For this review, take the finished solid that the model builds, in its own axes (mm). Face numbers are marked on the shaded views. A direction names the side the tool comes from. Round coordinates to 2 decimals unless told otherwise and drop trailing zeros. Order: outer loops, then holes, each group sorted by start corner. A loop starts at its lowest first (then second) coordinate and runs counter-clockwise, first axis right, second up. Notation, with made-up numbers: (-22.5, 55.5) - (13.5, 55.5) arc R34 ccw to (13.5, 85.5) - close; hole circle Ø10 at (33.5, 23.5). An arc over 180 degrees is marked (long way). One line per question, with ' | ' between items.
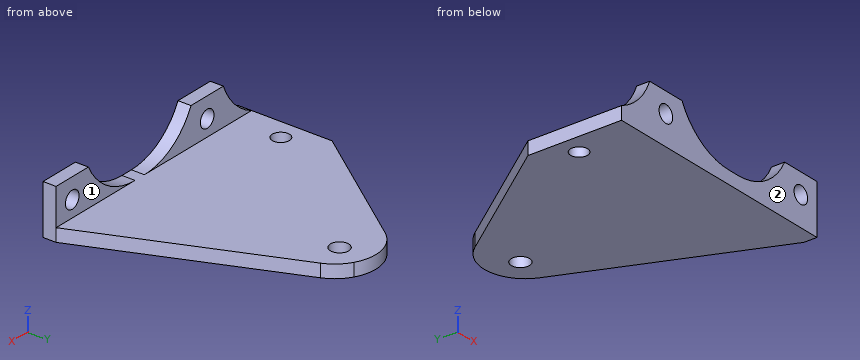
Autodesk Inventor part; units mm, degrees
ref_plane "YZ Plane" through (0, 0, 0) normal (1, 0, 0) x (0, 1, 0)
ref_plane "XZ Plane" through (0, 0, 0) normal (0, 1, 0) x (-1, 0, 0)
ref_plane "XY Plane" through (0, 0, 0) normal (0, 0, 1) x (1, 0, 0)
sketch "Эскиз1" plane through (0, 0, 0) normal (0, 0, 1) x (1, 0, 0)
  circle A0 centre (0, 0) radius 2.1
  line L0 (-5, 14.35) -> (5, 14.35)
  line L1 (5, 14.35) -> (5, -14.35)
  line L2 (5, -14.35) -> (-5, -14.35)
  line L3 (-5, -14.35) -> (-5, 14.35)
  line L4 (-5, 14.35) -> (5, -14.35) construction
  line L5 (5, 14.35) -> (-5, -14.35) construction
  line L6 (-5, 7) -> (5, 7)
  dimension "d0" = 4.2
  dimension "d2" = 10
  dimension "d3" = 28.7
  dimension "d4" = 7
extrude "Выдавливание1" add sketch "Эскиз1" along normal blind 3.2 contours L6 L1 L2 L3
sketch "Эскиз2" plane through (0, 0, 3.2) normal (0, 0, 1) x (1, 0, 0)
  line L0 (5, -14.35) -> (5, 7)
  line L1 (5, -14.35) -> (-5, -14.35)
  line L2 (-5, -14.35) -> (-5, -11.15)
  line L3 (-5, -11.15) -> (5, -11.15)
  line L4 (5, -11.15) -> (5, -14.35)
  point P0 (0, 0)
  point P1 (5, -11.15)
  dimension "d7" = 10
  dimension "d8" = 3.2
extrude "Выдавливание2" add sketch "Эскиз2" along normal blind 13
sketch "Эскиз3" plane through (-5, -11.15, 16.2) normal (0, 1, 0) x (1, 0, 0)
  line L0 (0, 10) -> (10, 10)
  line L1 (5, 10) -> (5, 0)
  line L2 (0, 0) -> (10, 0)
  circle A0 centre (5, 5) radius 2.1
  point P0 (5, 16.2)
  dimension "d12" = 4.2
extrude "Выдавливание3" cut sketch "Эскиз3" against normal blind 13
sketch "Эскиз4" plane through (0, 0, 3.2) normal (0, 0, 1) x (1, 0, 0)
  circle A0 centre (27.823512, 36.442015) radius 2.691667
  line L0 (25.598764, 34.926903) -> (0, 0)
  line L1 (17.757888, 39.624709) -> (-5, 8.573892)
  line L2 (-5, 7) -> (-5, -11.15)
  line L3 (-5, 7) -> (-5, 8.573892)
  line L4 (-5, -14.35) -> (5, -14.35)
  line L5 (5, -14.35) -> (5, -11.15)
  line L6 (5, -11.15) -> (-5, -11.15)
  line L7 (-5, -11.15) -> (-5, -14.35)
  line L8 (27.823512, 36.442015) -> (27.823512, -3.381482)
  line L9 (35.823512, 33.713219) -> (35.823512, -14.35)
  arc A1 (35.823512, 33.713219) -> (17.757888, 39.624709) centre (25.823512, 33.713219) ccw
  line L10 (-5, -14.35) -> (35.823512, -14.35)
  circle A2 centre (27.823512, 36.442015) radius 2.25
  line L11 (-5, 8.573892) -> (-5, -14.35)
  circle A3 centre (0, 0) radius 2.1
  point P0 (-5, -8.15)
  point P1 (-5, -11.15)
  dimension "d15" = 10
  dimension "d16" = 8
  dimension "d17" = 10
  dimension "d18" = 4.5
extrude "Выдавливание4" add sketch "Эскиз4" against normal up to surface (3.2 mm away) contours A0 | A1 L9 L10 L5 L6 L2 L3 L1
ref_plane "РабПлоскость1" through (20.202, -14.35, 16.2) normal (-1, 0, 0) x (0, 0, 1)
mirror "Зеркальное отражение1" about plane through (20.202, -14.35, 16.2) normal (-1, 0, 0) of "Выдавливание2", "Выдавливание3"
sketch "Эскиз6" plane through (0, 0, 0) normal (0, 0, -1) x (-1, 0, 0)
  circle A0 centre (-17.823512, 36.442015) radius 2.25
  circle A1 centre (10, 0) radius 2.1
  line L0 (5, -14.35) -> (-35.823512, -14.35)
  line L1 (5, -14.35) -> (5, 8.573892)
  line L2 (15, 8.573892) -> (-7.757888, 39.624709)
  arc A2 (-7.757888, 39.624709) -> (-25.823512, 33.713219) centre (-15.823512, 33.713219) ccw
  line L3 (-25.823512, 33.713219) -> (-25.823512, -14.35)
  circle A3 centre (-27.823512, 36.442015) radius 2.25
  circle A4 centre (0, 0) radius 2.1
  line L4 (5, -14.35) -> (-35.823512, -14.35)
  line L5 (5, -14.35) -> (5, 8.573892)
  line L6 (5, 8.573892) -> (-17.757888, 39.624709)
  arc A5 (-17.757888, 39.624709) -> (-35.823512, 33.713219) centre (-25.823512, 33.713219) ccw
  line L7 (-35.823512, 33.713219) -> (-35.823512, -14.35)
  line L8 (-35.823512, -14.35) -> (-35.823512, -11.15)
  line L9 (-35.823512, -11.15) -> (-45.404, -11.15)
  line L10 (-45.404, -11.15) -> (-45.404, -14.35)
  line L11 (-45.404, -14.35) -> (-35.823512, -14.35)
  line L12 (-25.823512, -14.35) -> (-45.404, -14.35)
  line L13 (0, 0) -> (10, 0)
  line L14 (15, 8.573892) -> (15, -18.0489)
  line L15 (-5, -14.35) -> (-35.404, -14.35)
  line L16 (-8, -14.35) -> (16.577235, -14.35)
  line L17 (-45.404, -11.15) -> (-35.708646, 35.224555)
  point P0 (-10, 0)
  point P1 (-20.823512, 42.373473)
  point P2 (15, -14.35)
  point P3 (-16.942673, 38.512431)
  point P4 (-15.583961, 36.658607)
  point P5 (5, 8.573892)
  dimension "d35" = 10
extrude "Выдавливание5" add sketch "Эскиз6" against normal up to surface (3.2 mm away) contours A0 L6 A5 A2 L2 L14 L16 L1 | A5 L7 L9 L17 | L9 L7 L11 L10
extrude "Выдавливание6" cut sketch "Эскиз6" against normal blind 10 contours A0 L6 | L6 A0 | A1
sketch "Эскиз7" plane through (0, 0, 3.2) normal (0, 0, 1) x (1, 0, 0)
  circle A0 centre (0, 0) radius 2.1
  line L0 (35.404, -14.35) -> (35.404, -11.15)
  line L1 (5, -14.35) -> (35.404, -14.35)
  arc A1 (35.708646, 35.224555) -> (20.823512, 42.373473) centre (25.823512, 33.713219) ccw
  line L2 (30.823512, 42.373473) -> (-5, -8.15)
  line L3 (35.404, -11.15) -> (45.404, -11.15)
  arc A2 (20.823512, 42.373473) -> (7.757888, 39.624709) centre (15.823512, 33.713219) ccw
  line L4 (-15, 8.573892) -> (7.757888, 39.624709)
  line L5 (-15, -14.35) -> (-15, 8.573892)
  line L6 (-5, -14.35) -> (-15, -14.35)
  line L7 (-5, -11.15) -> (-5, -14.35)
  circle A3 centre (17.823512, 36.442015) radius 2.25
  circle A4 centre (17.823512, 36.442015) radius 2.25
  circle A5 centre (27.823512, 36.442015) radius 2.25
  circle A6 centre (0, 0) radius 2.1
  circle A7 centre (-10, 0) radius 2.1
  line L8 (5, -14.35) -> (35.404, -14.35)
  line L9 (35.404, -14.35) -> (35.404, -11.15)
  line L10 (35.404, -11.15) -> (45.404, -11.15)
  arc A8 (35.708646, 35.224555) -> (20.823512, 42.373473) centre (25.823512, 33.713219) ccw
  arc A9 (20.823512, 42.373473) -> (7.757888, 39.624709) centre (15.823512, 33.713219) ccw
  line L11 (-15, 8.573892) -> (7.757888, 39.624709)
  line L12 (-15, -14.35) -> (-15, 8.573892)
  line L13 (-5, -14.35) -> (-15, -14.35)
  line L14 (-5, -11.15) -> (-5, -14.35)
  line L15 (35.708646, 35.224555) -> (45.404, -11.15)
  line L16 (35.708646, 35.224555) -> (45.404, -11.15)
  circle A10 centre (15.823537, 33.690994) radius 10.021745
  circle A11 centre (25.823512, 33.713219) radius 10
  line L17 (35.708646, 35.224555) -> (-5, 35.224555)
  line L18 (45.404, -11.15) -> (25.071691, 37.551955)
  line L19 (5, -14.35) -> (5, -11.15)
  line L20 (5, -14.35) -> (5, -11.15)
  line L21 (-5, -11.15) -> (5, -11.15)
  line L22 (-5, -11.15) -> (5, -11.15)
  point P0 (-0.639537, -2.000248)
  point P1 (1.675949, 1.265384)
  point P2 (20.826018, 42.374919)
extrude "Выдавливание7" add sketch "Эскиз7" against normal up to surface (3.2 mm away) contours A0 L2 | L2 A0 | L17 L18 L2 A5 | A5 L18 L17 | A5 L17 L18 | L2 L18 A5 | L17 A5 L2 L18 | L2 A5 L18
sketch "Эскиз7 outline for Выдавливание8" plane through (0, 0, 3.2) normal (0, 0, 1) x (1, 0, 0)
  arc A0 (35.708646, 35.224555) -> (20.826018, 42.374919) centre (25.823512, 33.713219) ccw
  line L0 (45.404, -11.15) -> (35.708646, 35.224555)
  line L1 (25.071691, 37.551955) -> (45.404, -11.15)
  arc A1 (20.826018, 42.374919) -> (25.071691, 37.551955) centre (15.823537, 33.690994) cw
extrude "Выдавливание8" cut sketch "Эскиз7 outline for Выдавливание8" against normal blind 10
sketch "Эскиз9" plane through (-5, -11.15, 16.2) normal (0, 1, 0) x (1, 0, 0)
  circle A0 centre (3.712, 5) radius 2.1
  line L0 (-1.288, 10) -> (8.712, 10)
  line L1 (-1.288, 10) -> (-1.288, 0)
  line L2 (8.712, 0) -> (-1.288, 0)
  line L3 (8.712, 13) -> (8.712, 0)
  line L4 (50.404, 13) -> (30.071691, 13)
  line L5 (30.071691, 13) -> (25.826018, 13)
  line L6 (25.826018, 13) -> (25.823512, 13)
  line L7 (12.757888, 13) -> (25.823512, 13)
  line L8 (-10, 13) -> (12.757888, 13)
  line L9 (0, 13) -> (-10, 13)
  line L10 (10, 13) -> (40.404, 13)
  line L11 (25.073512, 13) -> (20.573512, 13)
  line L12 (-7.1, 13) -> (-2.9, 13)
  line L13 (-1.288, 10) -> (-1.288, 15.274869)
  line L14 (0, 13) -> (0, 0)
  line L15 (0, 13) -> (0, 0)
  circle A1 centre (5, 5) radius 2.1
  line L16 (0, 13) -> (0, 0)
  line L17 (10, 0) -> (0, 0)
  line L18 (10, 13) -> (10, 0)
  line L19 (0, 13) -> (10, 13)
  line L20 (0, 13) -> (10, 13)
  line L21 (8.712, 10) -> (12.757888, 10)
  line L22 (3.712, 5) -> (3.712, 9)
  circle A2 centre (3.712, 9) radius 2.1
  line L23 (11.441296, 4) -> (-2.9, 4)
  line L24 (40.404, 13) -> (50.404, 13)
  point P0 (5, 16.2)
  point P1 (0, 10)
  point P2 (-1.288, 13)
  point P3 (0, 10)
  point P4 (-1.288, 4)
  point P5 (8.712, 4)
  dimension "d42" = 4
  dimension "d43" = 4.2
  dimension "d44" = 4
extrude "Выдавливание10" add sketch "Эскиз9" against normal up to surface (3.2 mm away) contours A0 L23 A1 | A0 A1 L23 | A1 L22 A2 A0 | A0 A2 L0 L3 L23 A1 | L23 A1 A0 | A0 A1 L23 | A2 L22 A0 | A0 A2 L0 | A1 L23 A0 A2 L22 | A1 L23 L3 L2 L14 A0 | A0 L23 A1 | L22 A2 A0 | L23 L14 L0 A2 A0 | L23 L1 L0 L14 | L14 L2 L1 L23 | L0 L13 L8 L14
extrude "Выдавливание11" cut sketch "Эскиз9" against normal blind 10 contours L23 A1 A0 | A0 A1 L23 | A2 L22 A0 | A0 A2 L0 | A1 L23 L3 L2 L14 A0 | A0 L23 A1 | L22 A2 A0 | L23 L18 L17 L3 | L3 L21 L18 L23 | L0 A2 | L14 L2 L1 L23 | L3 L8 L18 L21 picked at (6.324605, 3.867911) picked at (4.682533, 3.889371) picked at (2.387395, 3.867911)
ref_plane "РабПлоскость2" through (19.558, -14.35, 16.2) normal (-1, 0, 0) x (0, 0, 1)
mirror "Зеркальное отражение2" about plane through (19.558, -14.35, 16.2) normal (-1, 0, 0) of "Выдавливание11", "Выдавливание10"
fillet "Сопряжение5" radius 16 3 edges at (35.404, -12.75, 3.2) (3.712, -12.75, 3.2) (-6.288, -12.75, 3.2)
properties part number "мертвое колесо 3"
(1) For the marked faces 1 and 2, list the 3-axis set-ups (+Z, -Z, +X, -X, +Y, -Y) from which the entire face can be reached by the end or side of a thin tool; tool diameter is ignored.
Output values:
face 1: +Z, +X, -X, +Y | face 2: +Z, -Z, +X, -X, -Y
(2) We need section C-C on z = 7.2. State the section outline as (x, y) points.
Output values:
outline: (-9.36, -14.35) - (-3.39, -14.35) - (-3.39, -11.15) - (-9.36, -11.15) - close; (0.81, -14.35) - (7.52, -14.35) - (7.52, -11.15) - (0.81, -11.15) - close; (31.6, -14.35) - (38.3, -14.35) - (38.3, -11.15) - (31.6, -11.15) - close; (42.5, -14.35) - (45.4, -14.35) - (45.4, -11.15) - (42.5, -11.15) - close
(3) We need section B-B on y = 0. State the section outline as (x, z) points, plus the area to 3 significant figures.
Output values:
outline: (-15, 0) - (-12.1, 0) - (-12.1, 3.2) - (-15, 3.2) - close; (-7.9, 0) - (40.75, 0) - (40.75, 3.2) - (-7.9, 3.2) - close | area: 165 mm^2
(4) For probe 1 along Y at (x, z) = (4, 7.75); probe 2 along Z at (x, y) = (23, 23); probe 3 along X at (y, z) = (0, 2.1), list the stretches that pass through material, from the lowest coordinate up. Write a range as [from, to].
Output values:
probe 1: [-14.35, -11.15] | probe 2: [0, 3.2] | probe 3: [-15, -12.1], [-7.9, 40.75]
(5) We need section A-A on x = -10. State the section outline as (y, z) points.
Output values:
outline: (-14.35, 0) - (-2.1, 0) - (-2.1, 3.2) - (-11.15, 3.2) - (-11.15, 6.54) - (-14.35, 6.54) - close; (2.1, 0) - (15.4, 0) - (15.4, 3.2) - (2.1, 3.2) - close
(6) Insertion check: pin 1 (17.5 mm diameter, centred on x = 9, y = 17.5, fed in from +Z). The pin has a flat end and moves straight along its axis. Give the tip position at first contact, or say it passes through.
Output values:
pin 1: z = 3.2
(7) We need section D-D on x = 0. State the section outline as (y, z) points.
Output values:
outline: (-14.35, 0) - (29.04, 0) - (29.04, 3.2) - (-11.15, 3.2) - (-11.15, 5.54) - (-14.35, 5.54) - close; (-14.35, 8.86) - (-11.15, 8.86) - (-11.15, 12.2) - (-14.35, 12.2) - close
